Check sheet for the modelled part. Datum: model origin and axes. Units: mm. A direction names the side the tool comes from. Round coordinates to 2 decimals unless told otherwise and drop trailing zeros. Loops run counter-clockwise (first coordinate to the right, second up) from the corner with the lowest first, then second, coordinate; pieces in that order, holes last. Notation, with made-up numbers: (-8.5, 2.5) -> (14.5, 2.5) arc R25 cw to (14.5, 16.5) -> close; hole circle Ø4 at (13.25, -38.5). An arc over 180 degrees is marked (long way). Use one line per item in the form item = value. Start each with the question number.
(1) Draft check along Y on faces 1 (the cylindrical face through (0.1, 18.18, 6.4)), 2 (the cylindrical face through (30.998, -17.037, 1.056)), 3 (the flat face through (30.25, 0, 1)). Enter one of: released by +Y, released by -Y, zero draft, split by the parting line, or undercut.
(2) Sectioned sample at C-C (y = -11). Record the cut outline in (x, z), and give its area (3 significant figures).
(3) Sectioned sample at A-A (y = 0). Record the cut outline in (x, z), and give its area (3 significant figures).
(4) Set-up check for faces 4 (the flat face through (-29.5, 1, -1)), 5 (the cylindrical face through (-29.76, -3.4, 2.37)), 6 (the flat face through (0, -17.75, 1)): record each of +Z, -Z, +X, -X, +Y, -Y from which the full face is reachable in a straight line by a thin tool's end or side.
(5) Sectioned sample at B-B (z = -2). Record the cut outline in (x, y), and give its area (3 significant figures).
(6) Sectioned sample at D-D (x = -7). Record the cut outline in (y, z), and give its area (3 significant figures).
(7) Material ranges on probe 1 along X at (y, z) = (2, 0); probe 2 along Y at (x, z) = (-15, 4); probe 3 along Y at (x, z) = (7.5, -0.5), recorded low to high. Write a range as [from, to].
(8) Go/stop test with flat-tipped pins: pin 1 (0.6 mm diameter, centred on x = -30, z = 4, fed in from -Y); pin 2 (6.5 mm diameter, centred on x = 11, y = 9.5, fed in from -Z); pin 3 (1 mm diameter, centred on x = -30, y = 0.5, fed in from +Z). Record where each tip stops, or that it passes through.
from build123d import *

# Parameters (mm, degrees)
F0_W         = 62.5
F0_H         = 36.5
F0_W_2       = 58.5
F0_H_2       = 31.5
F1_DEPTH     = 7
F3_DEPTH     = 1.5
F4_W         = 62.5
F4_H         = 36.5
F5_DEPTH     = 3
F7_DEPTH     = 2.5
F8_R         = 2.5
F9_T1_DEPTH  = 57.5
F9_T3_DEPTH  = 31.5
F9_T6_ANGLE  = 90
F9_T8_ANGLE  = 90
F9_T10_ANGLE = 90
F9_T12_ANGLE = 90
F10_W        = 1.25
F10_H        = 8.5
F11_DEPTH    = 2


# Not quite as in the source:
# - a fillet or chamfer that OpenCascade refuses, or shapes differently, is made with other operations: its cross-section is extruded or revolved along the edge and cut away or added


with BuildPart() as f1:
    # F0 (on Top) → F1 (new body)
    with BuildSketch(Plane.XY):
        with Locations((0.5, 0.5)):
            Rectangle(F0_W, F0_H)
        with Locations((1, 0.5)):
            Rectangle(F0_W_2, F0_H_2, mode=Mode.SUBTRACT)
    extrude(amount=F1_DEPTH)

    # F2 (on face) → F3 (join)
    with BuildSketch(Plane.XY.offset(7)):
        Polygon((30.25, 16.25), (-28.25, 16.25), (-28.25, -15.25), (30.25, -15.25), (30.25, -6), (30.25, 7), align=None)
    extrude(amount=-F3_DEPTH)

    # F4 (on face) → F5 (join)
    with BuildSketch(Plane(origin=(0, 0, 0), x_dir=(1, 0, 0), z_dir=(0, 0, -1))):
        with Locations((0.5, -0.5)):
            Rectangle(F4_W, F4_H)
        Polygon((-29.5, -17.522141248), (-29.5, 16.5), (30.25, 16.5), (30.25, 15.25), (30.25, -16.25), (30.25, -17.522141248), align=None, mode=Mode.SUBTRACT)
    extrude(amount=F5_DEPTH)

    # F6 (on face) → F7 (cut)
    with BuildSketch(Plane.YZ.offset(-28.25)):
        with BuildLine():
            Line((4, 5.5), (-3, 5.5))
            ThreePointArc((-3, 5.5), (-3.5303300859, 5.2803300859), (-3.75, 4.75))
            Line((-3.75, 4.75), (-3.75, 3.5))
            ThreePointArc((-3.75, 3.5), (-3.1642135624, 2.0857864376), (-1.75, 1.5))
            Line((-1.75, 1.5), (2.75, 1.5))
            ThreePointArc((2.75, 1.5), (4.1642135624, 2.0857864376), (4.75, 3.5))
            Line((4.75, 3.5), (4.75, 4.75))
            ThreePointArc((4.75, 4.75), (4.5303300859, 5.2803300859), (4, 5.5))
        make_face()
    extrude(amount=-F7_DEPTH, mode=Mode.SUBTRACT)

    # F8
    f8_edges = [f1.edges().sort_by_distance(p)[0] for p in [
        (-30.75, 18.75, 2),
        (-30.75, -17.75, 2),
        (31.75, 18.75, 2),
        (31.75, -17.75, 2),
    ]]
    fillet(f8_edges, radius=F8_R)

    # F9: fillet of radius 2 on 8 edges, made by hand

    # F9_s2 → F9_t1 (cut)
    with BuildSketch(Plane.YZ.offset(-28.25)):
        with BuildLine():
            ThreePointArc((-15.75, 7), (-17.1642135624, 6.4142135624), (-17.75, 5))
            Line((-17.75, 5), (-17.75, 7))
            Line((-17.75, 7), (-15.75, 7))
        make_face()
        with BuildLine():
            ThreePointArc((18.75, 5), (18.1642135624, 6.4142135624), (16.75, 7))
            Line((16.75, 7), (18.75, 7))
            Line((18.75, 7), (18.75, 5))
        make_face()
    extrude(amount=F9_T1_DEPTH, mode=Mode.SUBTRACT)

    # F9_s4 → F9_t3 (cut)
    with BuildSketch(Plane.XZ.offset(-16.25)):
        with BuildLine():
            ThreePointArc((29.75, 7), (31.1642135624, 6.4142135624), (31.75, 5))
            Line((31.75, 5), (31.75, 7))
            Line((31.75, 7), (29.75, 7))
        make_face()
        with BuildLine():
            ThreePointArc((-28.75, 7), (-30.1642135624, 6.4142135624), (-30.75, 5))
            Line((-30.75, 5), (-30.75, 7))
            Line((-30.75, 7), (-28.75, 7))
        make_face()
    extrude(amount=F9_T3_DEPTH, mode=Mode.SUBTRACT)

    # F9_s5 → F9_t6 (revolve, cut)
    with BuildSketch(Plane.YZ.offset(29.25)):
        with BuildLine():
            ThreePointArc((16.75, 7), (18.1642135624, 6.4142135624), (18.75, 5))
            Line((18.75, 5), (18.75, 7))
            Line((18.75, 7), (16.75, 7))
        make_face()
    revolve(axis=Axis((29.25, 16.25, 7), (0, 0, -1)), revolution_arc=F9_T6_ANGLE, mode=Mode.SUBTRACT)

    # F9_s7 → F9_t8 (revolve, cut)
    with BuildSketch(Plane.YZ.offset(-28.25)):
        with BuildLine():
            ThreePointArc((16.75, 7), (18.1642135624, 6.4142135624), (18.75, 5))
            Line((18.75, 5), (18.75, 7))
            Line((18.75, 7), (16.75, 7))
        make_face()
    revolve(axis=Axis((-28.25, 16.25, 7), (0, 0, 1)), revolution_arc=F9_T8_ANGLE, mode=Mode.SUBTRACT)

    # F9_s9 → F9_t10 (revolve, cut)
    with BuildSketch(Plane.XZ.offset(15.25)):
        with BuildLine():
            ThreePointArc((29.75, 7), (31.1642135624, 6.4142135624), (31.75, 5))
            Line((31.75, 5), (31.75, 7))
            Line((31.75, 7), (29.75, 7))
        make_face()
    revolve(axis=Axis((29.25, -15.25, 7), (0, 0, -1)), revolution_arc=F9_T10_ANGLE, mode=Mode.SUBTRACT)

    # F9_s11 → F9_t12 (revolve, cut)
    with BuildSketch(Plane.XZ.offset(15.25)):
        with BuildLine():
            ThreePointArc((-28.75, 7), (-30.1642135624, 6.4142135624), (-30.75, 5))
            Line((-30.75, 5), (-30.75, 7))
            Line((-30.75, 7), (-28.75, 7))
        make_face()
    revolve(axis=Axis((-28.25, -15.25, 7), (0, 0, 1)), revolution_arc=F9_T12_ANGLE, mode=Mode.SUBTRACT)

    # F10 (on face) → F11 (cut)
    with BuildSketch(Plane(origin=(0, 0, 0), x_dir=(1, 0, 0), z_dir=(0, 0, -1))):
        with Locations((-28.875, -0.5)):
            Rectangle(F10_W, F10_H)
    extrude(amount=-F11_DEPTH, mode=Mode.SUBTRACT)


solid = f1.part
Checks:
q1.face_1 = released by +Y
q1.face_2 = released by -Y
q1.face_3 = undercut
q2.outline = (-30.75, -3) -> (-29.5, -3) -> (-29.5, 0) -> (-28.25, 0) -> (-28.25, 5.5) -> (30.25, 5.5) -> (30.25, -3) -> (31.75, -3) -> (31.75, 5) arc R2 ccw to (29.75, 7) -> (-28.75, 7) arc R2 ccw to (-30.75, 5) -> close
q2.area = 122 mm2
q3.outline = (-30.75, -3) -> (-29.5, -3) -> (-29.5, 1.5) -> (-30.75, 1.5) -> close; (-30.69, 5.5) -> (30.25, 5.5) -> (30.25, -3) -> (31.75, -3) -> (31.75, 5) arc R2 ccw to (29.75, 7) -> (-28.75, 7) arc R2 ccw to start
q3.area = 110 mm2
q4.face_4 = -Z
q4.face_5 = -X
q4.face_6 = +Z, -Z, +X, -X, -Y
q5.outline = (-30.75, -15.25) arc R2.5 ccw to (-28.25, -17.75) -> (29.25, -17.75) arc R2.5 ccw to (31.75, -15.25) -> (31.75, 16.25) arc R2.5 ccw to (29.25, 18.75) -> (-28.25, 18.75) arc R2.5 ccw to (-30.75, 16.25) -> close; hole (-29.5, -16.5) -> (30.25, -16.5) -> (30.25, 17.52) -> (-29.5, 17.52) -> close
q5.area = 243 mm2
q6.outline = (-17.75, -3) -> (-16.5, -3) -> (-16.5, 0) -> (-15.25, 0) -> (-15.25, 5.5) -> (16.25, 5.5) -> (16.25, 0) -> (17.52, 0) -> (17.52, -3) -> (18.75, -3) -> (18.75, 5) arc R2 ccw to (16.75, 7) -> (-15.75, 7) arc R2 ccw to (-17.75, 5) -> close
q6.area = 88.0 mm2
q7.probe_1 = [-30.75, -29.5], [30.25, 31.75]
q7.probe_2 = [-17.75, -15.25], [16.25, 18.75]
q7.probe_3 = [-17.75, -16.5], [17.52, 18.75]
q8.pin_1 = -17.29
q8.pin_2 = 5.5
q8.pin_3 = 6.85
